Check sheet for the modelled part. Datum: model origin and axes. Units: mm. A direction names the side the tool comes from. Coordinates: 2 decimals unless noted, no trailing zeros. Order: outer loops, then holes, each group sorted by start corner. A loop starts at its lowest first (then second) coordinate and runs counter-clockwise, first axis right, second up.
1. Thickness scan on line 1 (Z direction, x = 9, y = -717); line 2 (X direction, y = -454, z = 62). Record the ranges inside material, lowest first.
2. Cross-section at B-B (z = 10). Enter the section's corners in (x, y).
3. Gauge pin test, flat end, axial feed: pin 1 Ø8 at (x, z) = (17.5, 45) entering from -Y. Record the tip position at first contact, or that the pin passes through.
4. Set-up check for faces 1 (the flat face through (13, -466, 76.2)), 2 (the flat face through (13, -466, 74.676)): record each of +Z, -Z, +X, -X, +Y, -Y from which the full face is reachable in a straight line by a thin tool's end or side.
5. Cross-section at C-C (y = -93). Enter the section's corners in (x, z).
6. Draft check along X on faces 3 (the flat face through (25.4, -466, 38)), 4 (the flat face through (1.524, -466, 38)), 5 (the flat face through (13, -466, 0)). Enter one of: released by +X, released by -X, zero draft, split by the parting line, or undercut.
7. Cross-section at A-A (x = 16.5). Enter the section's corners in (y, z), then the cut area to 3 significant figures.
```python
from build123d import *

# Parameters (mm, degrees)
F1_DEPTH = 946.15


# Not quite as in the source:
# - a feature names something its author has since deleted; it is built from what else it names


with BuildPart() as f1:
    # F0 (on Front) → F1 (new body)
    with BuildSketch(Plane.XZ):
        with BuildLine():
            ThreePointArc((0, 1.651), (0.4835667043, 0.4835667043), (1.651, 0))
            Line((1.651, 0), (23.749, 0))
            ThreePointArc((23.749, 0), (24.9164332957, 0.4835667043), (25.4, 1.651))
            Line((25.4, 1.651), (25.4, 74.549))
            ThreePointArc((25.4, 74.549), (24.9164332957, 75.7164332957), (23.749, 76.2))
            Line((23.749, 76.2), (1.651, 76.2))
            ThreePointArc((1.651, 76.2), (0.4835667043, 75.7164332957), (0, 74.549))
            Line((0, 74.549), (0, 1.651))
        make_face()
        with BuildLine():
            ThreePointArc((1.5240004182, 74.549), (1.5611977345, 74.6388022655), (1.651, 74.6759995818))
            Line((1.651, 74.6759995818), (23.749, 74.6759995818))
            ThreePointArc((23.749, 74.6759995818), (23.8388022655, 74.6388022655), (23.8759995818, 74.549))
            Line((23.8759995818, 74.549), (23.8759995818, 1.651))
            ThreePointArc((23.8759995818, 1.651), (23.8388022655, 1.5611977345), (23.749, 1.5240004182))
            Line((23.749, 1.5240004182), (1.651, 1.5240004182))
            ThreePointArc((1.651, 1.5240004182), (1.5611977345, 1.5611977345), (1.5240004182, 1.651))
            Line((1.5240004182, 1.651), (1.5240004182, 74.549))
        make_face(mode=Mode.SUBTRACT)
    extrude(amount=F1_DEPTH)


solid = f1.part
```
Data:
1. line 1: z = 0 to 1.52, 74.68 to 76.2
1. line 2: x = 0 to 1.52, 23.88 to 25.4
2. outline: (0, -946.15) - (1.52, -946.15) - (1.52, 0) - (0, 0) - close; (23.88, -946.15) - (25.4, -946.15) - (25.4, 0) - (23.88, 0) - close
3. pin 1: passes through
4. face 1: +Z, +X, -X, +Y, -Y
4. face 2: +Y, -Y
5. outline: (0, 1.65) arc R1.65 ccw to (1.65, 0) - (23.75, 0) arc R1.65 ccw to (25.4, 1.65) - (25.4, 74.55) arc R1.65 ccw to (23.75, 76.2) - (1.65, 76.2) arc R1.65 ccw to (0, 74.55) - close; hole (1.52, 1.65) arc R0.13 ccw to (1.65, 1.52) - (23.75, 1.52) arc R0.13 ccw to (23.88, 1.65) - (23.88, 74.55) arc R0.13 ccw to (23.75, 74.68) - (1.65, 74.68) arc R0.13 ccw to (1.52, 74.55) - close
6. face 3: released by +X
6. face 4: undercut
6. face 5: zero draft
7. outline: (-946.15, 0) - (0, 0) - (0, 1.52) - (-946.15, 1.52) - close; (-946.15, 74.68) - (0, 74.68) - (0, 76.2) - (-946.15, 76.2) - close
7. area: 2,880 mm2
